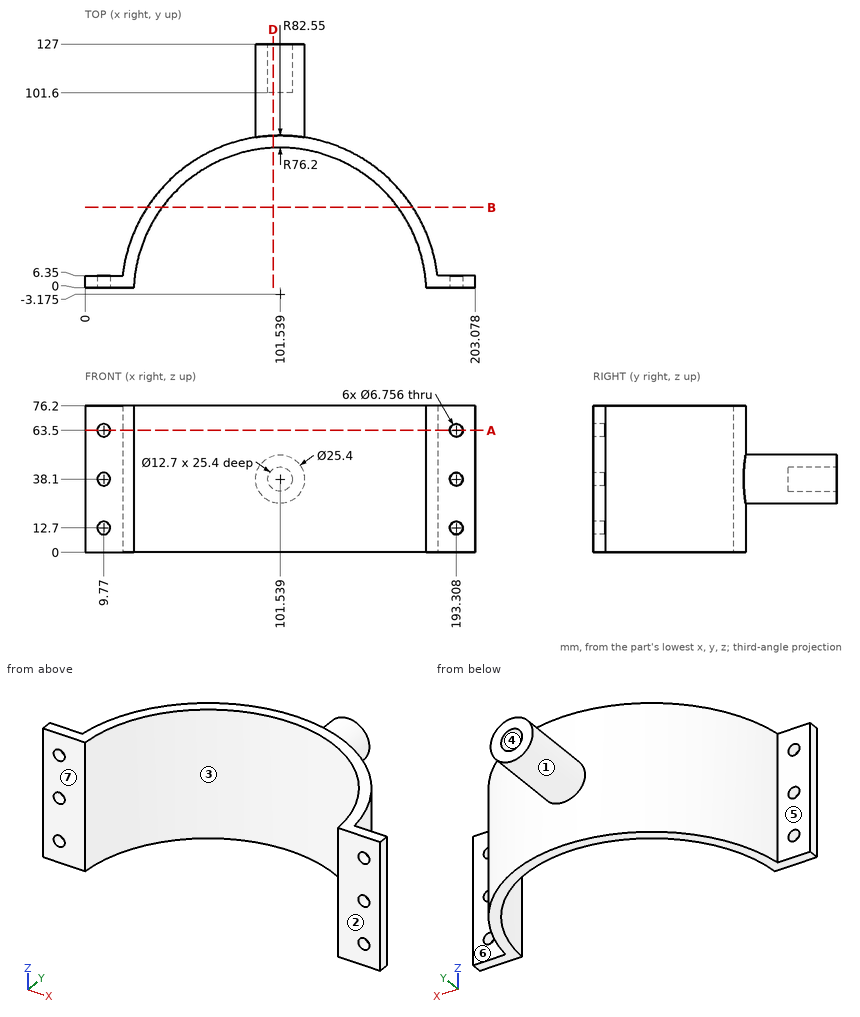
Answer from the drawing. Dimensions are ordinates in mm from the lowest x, y and z of the part. A direction names the side the tool comes from. Give positions to 0.01 mm unless a question says otherwise; leave off trailing zeros. Loops run counter-clockwise (first coordinate to the right, second up) from the corner with the lowest first, then second, coordinate; pieces in that order, holes last.
Item 1: For the marked faces 5, 6 and 7, determine the directions among +Z, -Z, +X, -X, +Y, -Y from which every point of the face is accessible in a straight line to the end or side of a thin tool.
Item 2: The part is cut by section B-B (y = 42). Write down the section's boundary in (x, z).
Item 3: Find the intervals of material crossed by line 1 along X through (y, z) = (2.25, 63.5) (1 decimal); line 2 along X through (y, z) = (3.5, 38.1) (1 decimal); line 3 along Y through (x, z) = (187, 33.5), in increasing order.
Item 4: The part is cut by section D-D (x = 98). Write down the section's boundary in (y, z), and give its area (3 significant figures).
Item 5: The mould has two halves that part along X. Classify the marked faces 1, 2, 3 and 4: released by +X, released by -X, zero draft, split by the parting line, or undercut.
Item 6: The part is cut by section A-A (z = 63.5). Give the number of separate pieces and of enclosed holes in the cut face, and give its area (3 significant figures).
Item 7: Each of these flat-tipped pins is pushed along its axis until it touches: pin 1 Ø4 at (x, z) = (9.77, 12.7) entering from +Y; pin 2 Ø15.5 at (x, z) = (8.5, 33) entering from +Y; pin 3 Ø3 at (y, z) = (65, 36) entering from -X; pin 4 Ø4 at (y, z) = (45.5, 49.5) entering from +X. Where does it stop, or does it pass through?
Taken from the geometry:
1. face 5: +Z, -Z, -X, +Y
1. face 6: +Z, -Z, +X, +Y
1. face 7: +Z, -Z, +X, -X, -Y
2. outline: (32.45, 0) - (40.17, 0) - (40.17, 76.2) - (32.45, 76.2) - close; (162.9, 0) - (170.63, 0) - (170.63, 76.2) - (162.9, 76.2) - close
3. line 1: x = 0 to 6.4, 13.1 to 25.5, 177.5 to 189.9, 196.7 to 203.1
3. line 2: x = 0 to 6.4, 13.1 to 25.6, 177.4 to 189.9, 196.7 to 203.1
3. line 3: y = 0 to 6.35
4. outline: (72.94, 0) - (79.3, 0) - (79.3, 25.9) - (127, 25.9) - (127, 32.83) - (101.6, 32.83) - (101.6, 43.37) - (127, 43.37) - (127, 50.3) - (79.3, 50.3) - (79.3, 76.2) - (72.94, 76.2) - close
4. area: 1,380 mm2
5. face 1: split by the parting line
5. face 2: zero draft
5. face 3: undercut
5. face 4: undercut
6. separate pieces: 3
6. enclosed holes: 0
6. area: 1,700 mm2
7. pin 1: passes through
7. pin 2: stops at y = 6.35
7. pin 3: stops at x = 52.87
7. pin 4: stops at x = 169.63
